Build history of the part. All positions in model axes, mm. Give positions to 0.01 mm unless a question says otherwise; leave off trailing zeros. Loops run counter-clockwise (first coordinate to the right, second up) from the corner with the lowest first, then second, coordinate; pieces in that order, holes last.
1) Band-saw the part on D-D on x = 43.5. List the corners of the cut face in (y, z) (3 decimals).
2) Wall check: line 1 (Y direction, x = 0, z = 2.25); line 2 (Y direction, x = 108, z = 1.5); line 3 (X direction, y = 0.5, z = 0.5). Give the ranges that are in metal, low to high.
3) Flat gauge pins, fed straight in: P1, Ø1.5, axis at y = -8.5, z = 1.5, coming from the -X side; P2, Ø2, axis at x = 65, z = 2.5, coming from the -Y side; P3, Ø2, axis at y = 8, z = 2, coming from the +X side. Where does each tip first touch, or does it go through?
4) Two-plate mould, pull along X, no slides. Class faces 1 (the flat face through (29, 0, 6.2)), 2 (the cylindrical face through (0, 8, 3)), 3 (the flat face through (11.53, -28.82, 3.06)): +X half, -X half, draft (parallel to the pull), parting line (faces both ways), or undercut.
5) Band-saw the part on C-C on z = 4.75. List the corners of the cut face in (x, y).
6) Band-saw the part on B-B on y = -4.75. List the corners of the cut face in (x, z).
7) Band-saw the part on A-A on x = 108. List the corners of the cut face in (y, z).
```python
from build123d import *

# Parameters (mm, degrees)
SKETCH1_R           = 2.5
SKETCH1_R_2         = 6.5
BOSS_EXTRUDE1_DEPTH = 6.2
CUT_EXTRUDE1_REACH  = 130.699
SKETCH2_R           = 1.5


with BuildPart() as part:
    # Sketch1 → Boss-Extrude1 (new body)
    with BuildSketch(Plane.XY):
        with BuildLine():
            Line((3.611111111, -29.781871609), (19.668670355, -27.834860643))
            ThreePointArc((19.668670355, -27.834860643), (27.894571922, -24.919368692), (34.095743926, -18.778439145))
            ThreePointArc((34.095743926, -18.778439145), (63.437182893, -0.609540518), (96, -12.041594579))
            ThreePointArc((96, -12.041594579), (123.291552208, -7.427545426), (110.046296296, 16.876393912))
            Line((110.046296296, 16.876393912), (3.611111111, 29.781871609))
            ThreePointArc((3.611111111, 29.781871609), (-30, 0), (3.611111111, -29.781871609))
        make_face()
        with Locations(Location((108, 0, 0), (0, 0, 180))):
            Circle(SKETCH1_R, mode=Mode.SUBTRACT)
        with Locations(Location((0, 0, 0), (0, 0, 180))):
            Circle(SKETCH1_R_2, mode=Mode.SUBTRACT)
    extrude(amount=BOSS_EXTRUDE1_DEPTH)

    # Sketch2 → Cut-Extrude1 (cut, up to next)
    with BuildSketch(Plane(origin=(0, 0, 0), x_dir=(-1, 0, 0), z_dir=(0, 0, -1)), mode=Mode.PRIVATE) as cut_extrude1_sk1:
        with Locations((8.227241336, -4.75)):
            Circle(SKETCH2_R)
    cut_extrude1_tool1 = extrude(cut_extrude1_sk1.sketch, amount=-CUT_EXTRUDE1_REACH, mode=Mode.PRIVATE) & part.part
    # Sketch2 → Cut-Extrude1 (cut, up to next)
    with BuildSketch(Plane(origin=(0, 0, 0), x_dir=(-1, 0, 0), z_dir=(0, 0, -1)), mode=Mode.PRIVATE) as cut_extrude1_sk2:
        with Locations((-8.227241336, -4.75)):
            Circle(SKETCH2_R)
    cut_extrude1_tool2 = extrude(cut_extrude1_sk2.sketch, amount=-CUT_EXTRUDE1_REACH, mode=Mode.PRIVATE) & part.part
    # Sketch2 → Cut-Extrude1 (cut, up to next)
    with BuildSketch(Plane(origin=(0, 0, 0), x_dir=(-1, 0, 0), z_dir=(0, 0, -1)), mode=Mode.PRIVATE) as cut_extrude1_sk3:
        with Locations((0, 9.5)):
            Circle(SKETCH2_R)
    cut_extrude1_tool3 = extrude(cut_extrude1_sk3.sketch, amount=-CUT_EXTRUDE1_REACH, mode=Mode.PRIVATE) & part.part
    add(cut_extrude1_tool1.solids().sort_by_distance((-8.227241, -4.75, 0))[0], mode=Mode.SUBTRACT)
    add(cut_extrude1_tool2.solids().sort_by_distance((8.227241, -4.75, 0))[0], mode=Mode.SUBTRACT)
    add(cut_extrude1_tool3.solids().sort_by_distance((0, 9.5, 0))[0], mode=Mode.SUBTRACT)


solid = part.part
```
Findings below:
1. outline: (-8.575, 0) - (24.945, 0) - (24.945, 6.2) - (-8.575, 6.2) - close
2. line 1: y = -30 to -6.5, 6.5 to 8, 11 to 30
2. line 2: y = -17 to -2.5, 2.5 to 17.12
2. line 3: x = -30 to -6.48, 6.48 to 105.55, 110.45 to 124.99
3. P1: stops at x = -28.98
3. P2: stops at y = -0.55
3. P3: stops at x = 123.49
4. face 1: draft
4. face 2: undercut
4. face 3: +X half
5. outline: (3.61, -29.78) - (19.67, -27.83) arc R20 ccw to (34.1, -18.78) arc R40 cw to (96, -12.04) arc R17 ccw (long way) to (110.05, 16.88) - (3.61, 29.78) arc R30 ccw (long way) to start; hole circle Ø3 at (-8.23, -4.75); hole circle Ø13 at (0, 0); hole circle Ø3 at (0, 9.5); hole circle Ø3 at (8.23, -4.75); hole circle Ø5 at (108, 0)
6. outline: (-29.62, 0) - (-9.73, 0) - (-9.73, 6.2) - (-29.62, 6.2) - close; (-6.73, 0) - (-4.44, 0) - (-4.44, 6.2) - (-6.73, 6.2) - close; (4.44, 0) - (6.73, 0) - (6.73, 6.2) - (4.44, 6.2) - close; (9.73, 0) - (49.57, 0) - (49.57, 6.2) - (9.73, 6.2) - close; (85.95, 0) - (124.32, 0) - (124.32, 6.2) - (85.95, 6.2) - close
7. outline: (-17, 0) - (-2.5, 0) - (-2.5, 6.2) - (-17, 6.2) - close; (2.5, 0) - (17.12, 0) - (17.12, 6.2) - (2.5, 6.2) - close
